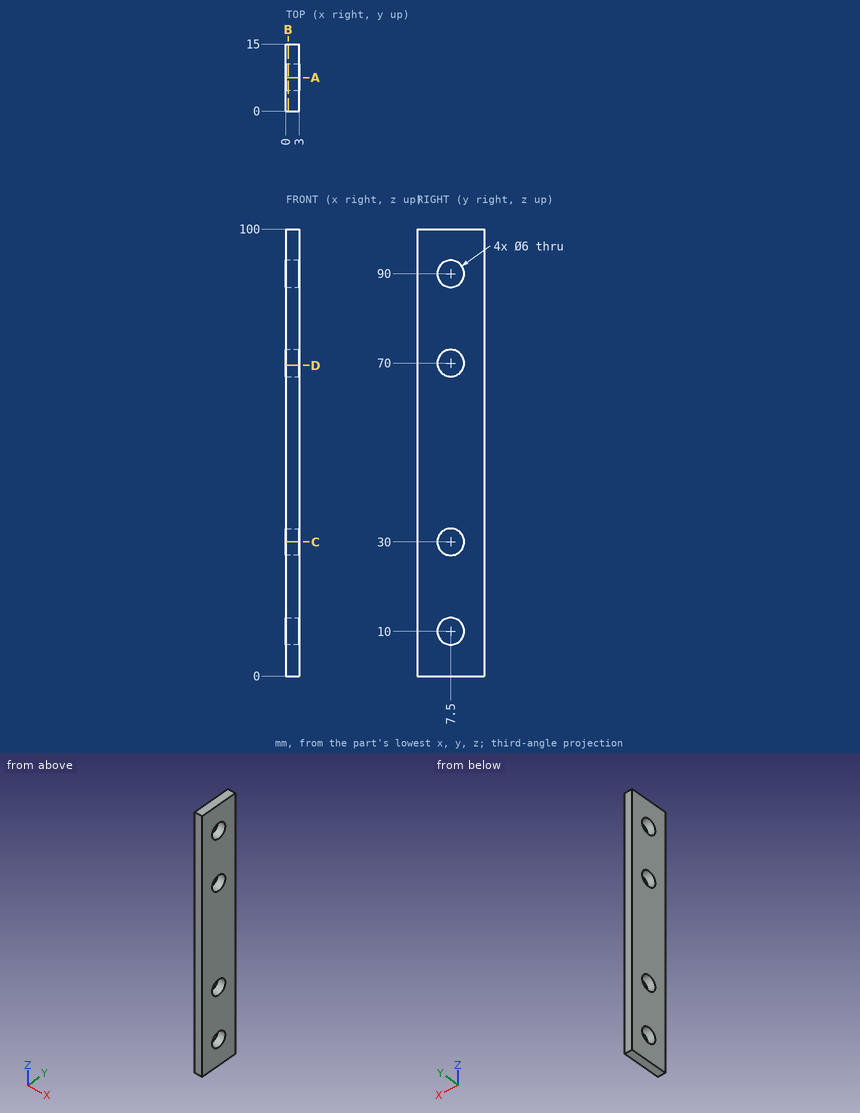
The figure shows three views and two pictorial views of one solid part (mm, origin at its lowest corner). Answer the questions. Round coordinates to 2 decimals unless told otherwise and drop trailing zeros. Order: outer loops, then holes, each group sorted by start corner. A loop starts at its lowest first (then second) coordinate and runs counter-clockwise, first axis right, second up. Notation, with made-up numbers: (25.25, 14) - (59.25, 14) arc R11 ccw to (59.25, 25) - close; hole circle Ø1 at (-22, 36.5). An arc over 180 degrees is marked (long way). Write item = value, one per line. Start each with the question number.
1) Section C-C, the plane z = 30 is taken. Write down the section's boundary in (x, y).
2) Straight lines are drawn through the part: L1, parallel to Y at x = 1, z = 90; L2, parallel to Z at x = 2.6, y = 8.75. For each, find the intervals that lie inside material, in ascending order.
3) Section A-A, the plane y = 7.5 is taken. Write down the section's boundary in (x, z), plus the area to 3 significant figures.
4) Section B-B, the plane x = 0.5 is taken. Write down the section's boundary in (y, z), plus the area to 3 significant figures.
5) Section D-D, the plane z = 69.5 is taken. Write down the section's boundary in (x, y).
Results list:
q1.outline = (0, 0) - (3, 0) - (3, 4.5) - (0, 4.5) - close; (0, 10.5) - (3, 10.5) - (3, 15) - (0, 15) - close
q2.L1 = 0 to 4.5, 10.5 to 15
q2.L2 = 0 to 7.27, 12.73 to 27.27, 32.73 to 67.27, 72.73 to 87.27, 92.73 to 100
q3.outline = (0, 0) - (3, 0) - (3, 7) - (0, 7) - close; (0, 13) - (3, 13) - (3, 27) - (0, 27) - close; (0, 33) - (3, 33) - (3, 67) - (0, 67) - close; (0, 73) - (3, 73) - (3, 87) - (0, 87) - close; (0, 93) - (3, 93) - (3, 100) - (0, 100) - close
q3.area = 228 mm^2
q4.outline = (0, 0) - (15, 0) - (15, 100) - (0, 100) - close; hole circle Ø6 at (7.5, 10); hole circle Ø6 at (7.5, 30); hole circle Ø6 at (7.5, 70); hole circle Ø6 at (7.5, 90)
q4.area = 1,390 mm^2
q5.outline = (0, 0) - (3, 0) - (3, 4.54) - (0, 4.54) - close; (0, 10.46) - (3, 10.46) - (3, 15) - (0, 15) - close
